```python
from build123d import *

# Parameters (mm, degrees)
SKETCH1_W           = 3.479672363
SKETCH1_H           = 4.175606835
SKETCH1_W_2         = 3.333333333
SKETCH1_H_2         = 4
BOSS_EXTRUDE1_DEPTH = 4
CAVITY1_START       = -27.230031218
CAVITY1_OUTLINE_W   = 16.666666667
CAVITY1_OUTLINE_H   = 4
CAVITY1_DEPTH       = 4


# Read off the part's stored shape, not the designer's step: Cavity1
with BuildPart() as part:
    # Sketch1 → Boss-Extrude1 (new body)
    with BuildSketch(Plane.XY):
        with Locations((-32.230031219, -14.092199994)):
            Rectangle(SKETCH1_W, SKETCH1_H)
        Polygon((-33.9698674, -20.355610246), (-33.9698674, -16.180003411), (-37.230031218, -16.180003411), (-37.230031218, -66.180003411), (-33.896697885, -66.180003411), (-33.896697885, -62.180003411), (-30.563364552, -62.180003411), (-30.563364552, -66.180003411), (-27.230031218, -66.180003411), (-27.230031218, -16.180003411), (-30.490195037, -16.180003411), (-30.490195037, -20.355610246), align=None)
        with Locations((-32.230031219, -18.267806828)):
            Rectangle(SKETCH1_W, SKETCH1_H)
        Polygon((-23.230031218, -16.180335931), (-27.230031218, -16.180003411), (-27.230031218, -66.180003411), (-23.230031218, -66.180003411), align=None)
        with Locations((-32.230031219, -64.180003411)):
            Rectangle(SKETCH1_W_2, SKETCH1_H_2)
        with Locations((-32.230031219, -68.180003411)):
            Rectangle(SKETCH1_W_2, SKETCH1_H_2)
    extrude(amount=BOSS_EXTRUDE1_DEPTH)

    # Cavity1 outline → Cavity1 (cut)
    with BuildSketch(Plane.YZ.offset(CAVITY1_START)):
        with Locations((-41.180335932, 2)):
            Rectangle(CAVITY1_OUTLINE_W, CAVITY1_OUTLINE_H)
    extrude(amount=CAVITY1_DEPTH, mode=Mode.SUBTRACT)


solid = part.part
```
Here's how the part is built. I have some questions about the finished solid (model axes, mm). A direction names the side the tool comes from. Coordinates: 2 decimals unless noted, no trailing zeros. Write each loop counter-clockwise with the first axis right and the second up, starting at its lowest first coordinate (ties: lowest second). Pieces come first, ordered by that corner, then holes. Notation, with made-up numbers: (34.5, -37.5) - (47.5, -37.5) arc R26 ccw to (47.5, -7.5) - close; hole circle Ø6 at (83, 4). An arc over 180 degrees is marked (long way). One line per item, written item: value.
1) On a 3-axis mill with a long thin cutter (end or side, diameter ignored), from which of +Z, -Z, +X, -X, +Y, -Y can I reach the whole of each face in a straight line? I mean faces 5 (the flat face through (-33.97, -14, 2)), 6 (the flat face through (-33.897, -68, 2)), 7 (the flat face through (-30.563, -68, 2)), 8 (the flat face through (-25, -32.847, 2)). Say none if no direction works.
Model answer:
face 5: +Z, -Z, -X, +Y
face 6: +Z, -Z, -X, -Y
face 7: +Z, -Z, +X, -Y
face 8: +Z, -Z, +X
2) Suppose I cut it at C-C on x = -27.75. Write out the boundary of the cut face in (y, z), and give its area (3 significant figures).
Model answer:
outline: (-66.18, 0) - (-16.18, 0) - (-16.18, 4) - (-66.18, 4) - close
area: 200 mm²
3) Suppose I cut it at B-B on y = -38.5. Write out the boundary of the cut face in (x, z), and give its area (3 significant figures).
Model answer:
outline: (-37.23, 0) - (-27.23, 0) - (-27.23, 4) - (-37.23, 4) - close
area: 40.0 mm²
4) Suppose I cut it at A-A on z = 1.05. Write out the boundary of the cut face in (x, y).
Model answer:
outline: (-37.23, -66.18) - (-33.9, -66.18) - (-33.9, -70.18) - (-30.56, -70.18) - (-30.56, -66.18) - (-23.23, -66.18) - (-23.23, -49.51) - (-27.23, -49.51) - (-27.23, -32.85) - (-23.23, -32.85) - (-23.23, -16.18) - (-27.23, -16.18) - (-30.49, -16.18) - (-30.49, -12) - (-33.97, -12) - (-33.97, -16.18) - (-37.23, -16.18) - close
5) We'd pull the mould along Y, two halves only. Please class faces 1 (the flat face through (-25, -49.514, 2)), 2 (the flat face through (-32, -41, 4)), 3 (the flat face through (-27.23, -41, 2)), 4 (the flat face through (-32, -70.18, 2)): pulls with the +Y half, pulls with the -Y half, needs draft (parallel to the pull), parting line crosses it, or undercut.
Model answer:
face 1: undercut
face 2: needs draft
face 3: undercut
face 4: pulls with the -Y half
6) I need wall thicknesses on line 1 along Y through (x, z) = (-34.25, 2.4); line 2 along X through (y, z) = (-14.5, 0.7); line 3 along Y through (x, z) = (-25, 3.8). Which ranges of each line are inside material? Lowest first, please.
Model answer:
line 1: y = -66.18 to -16.18
line 2: x = -33.97 to -30.49
line 3: y = -66.18 to -49.51, -32.85 to -16.18
7) I'm going to push flat-ended pins straight in: P1, Ø5, axis at x = -28.5, y = -46.5, coming from the -Z side; P2, Ø2, axis at y = -68, z = 3, coming from the +X side; P3, Ø2, axis at y = -13.5, z = 3, coming from the -X side; P4, Ø1.2, axis at x = -28.5, z = 2.5, coming from the -Y side. Where does each tip first touch, or does it pass through?
Model answer:
P1: stops at z = 0
P2: stops at x = -30.56
P3: stops at x = -33.97
P4: stops at y = -66.18
